from build123d import *

# Parameters (mm, degrees)
SKETCH1_W               = 110
SKETCH1_H               = 70
BOSS_EXTRUDE1_DEPTH     = 7
FILLET1_R               = 5
CUT_EXTRUDE1_DEPTH      = 40
SHELL1_START            = 5
SHELL1_DEPTH            = 2
SHELL1_START_2          = 2
SHELL1_2_DEPTH          = 3
SHELL1_START_3          = -42
SHELL1_3_DEPTH          = 40
SHELL1_4_DEPTH          = 2
SKETCH2_W               = 80
SKETCH2_H               = 0.8
SKETCH2_W_2             = 0.8
SKETCH2_H_2             = 40
BOSS_EXTRUDE2_DEPTH     = 6
CHAMFER1_SIZE           = 0.5
SKETCH8_R               = 4.15
BOSS_EXTRUDE3_DEPTH     = 3.2
CUT_EXTRUDE5_DEPTH      = 131.48770057
CUT_EXTRUDE5_DEPTH_BACK = 131.48770057
SKETCH9_R               = 1.5
SKETCH10_R              = 3
CUT_EXTRUDE6_DEPTH      = 3.2
CHAMFER2_SIZE           = 0.5
BOSS_EXTRUDE4_REACH     = 120.017


with BuildPart() as part:
    # Sketch1 → Boss-Extrude1 (new body)
    with BuildSketch(Plane(origin=(0, 0, 0), x_dir=(1, 0, 0), z_dir=(0, 1, 0))):
        with Locations((55, 35)):
            Rectangle(SKETCH1_W, SKETCH1_H)
    extrude(amount=BOSS_EXTRUDE1_DEPTH)

    # Fillet1
    fillet1_edges = [part.edges().sort_by_distance(p)[0] for p in [
        (0, 3.5, -70),
        (110, 3.5, -70),
        (110, 3.5, 0),
        (0, 3.5, 0),
    ]]
    fillet(fillet1_edges, radius=FILLET1_R)

    # Sketch3 → Cut-Extrude1 (cut)
    with BuildSketch(Plane.XY):
        Polygon((38, 0), (35, 3), (45, 3), (42, 0), align=None)
        Polygon((68, 0), (65, 3), (75, 3), (72, 0), align=None)
    extrude(amount=-CUT_EXTRUDE1_DEPTH, mode=Mode.SUBTRACT)

    # Shell1: read off the stored shape, not the designer's step
    # Shell1 outline → Shell1 (cut)
    with BuildSketch(Plane(origin=(0, 0, 0), x_dir=(1, 0, 0), z_dir=(0, 1, 0)).offset(SHELL1_START)):
        with BuildLine():
            Line((2, 65), (2, 5))
            ThreePointArc((2, 5), (2.878679656, 2.878679656), (5, 2))
            Line((5, 2), (105, 2))
            ThreePointArc((105, 2), (107.121320344, 2.878679656), (108, 5))
            Line((108, 5), (108, 65))
            ThreePointArc((108, 65), (107.121320344, 67.121320344), (105, 68))
            Line((105, 68), (5, 68))
            ThreePointArc((5, 68), (2.878679656, 67.121320344), (2, 65))
        make_face()
    extrude(amount=SHELL1_DEPTH, mode=Mode.SUBTRACT)

    # Shell1 2 outline → Shell1 2 (cut)
    with BuildSketch(Plane(origin=(0, 0, 0), x_dir=(1, 0, 0), z_dir=(0, 1, 0)).offset(SHELL1_START_2)):
        with BuildLine():
            Line((2, 65), (2, 5))
            ThreePointArc((2, 5), (2.878679656, 2.878679656), (5, 2))
            Line((5, 2), (105, 2))
            ThreePointArc((105, 2), (107.121320344, 2.878679656), (108, 5))
            Line((108, 5), (108, 65))
            ThreePointArc((108, 65), (107.121320344, 67.121320344), (105, 68))
            Line((105, 68), (5, 68))
            ThreePointArc((5, 68), (2.878679656, 67.121320344), (2, 65))
        make_face()
    extrude(amount=SHELL1_2_DEPTH, mode=Mode.SUBTRACT)

    # Shell1 3 outline → Shell1 3 (add)
    with BuildSketch(Plane.XY.offset(SHELL1_START_3)):
        Polygon((36, 2), (35, 3), (45, 3), (44, 2), (46.828427125, 2), (49.828427125, 5), (30.171572875, 5), (33.171572875, 2), align=None)
        Polygon((60.171572875, 5), (63.171572875, 2), (66, 2), (65, 3), (75, 3), (74, 2), (76.828427125, 2), (79.828427125, 5), align=None)
    extrude(amount=SHELL1_3_DEPTH)

    # Shell1 4 outline → Shell1 4 (add)
    with BuildSketch(Plane.XY.offset(SHELL1_START_3)):
        Polygon((45, 3), (35, 3), (36, 2), (44, 2), align=None)
        Polygon((65, 3), (66, 2), (74, 2), (75, 3), align=None)
    extrude(amount=SHELL1_4_DEPTH)

    # Sketch2 → Boss-Extrude2 (add)
    with BuildSketch(Plane(origin=(0, 2, 0), x_dir=(1, 0, 0), z_dir=(0, 1, 0))):
        with Locations((55, 67.6)):
            Rectangle(SKETCH2_W, SKETCH2_H)
        with Locations((107.6, 35)):
            Rectangle(SKETCH2_W_2, SKETCH2_H_2)
        with Locations((2.4, 35)):
            Rectangle(SKETCH2_W_2, SKETCH2_H_2)
    extrude(amount=BOSS_EXTRUDE2_DEPTH)

    # Chamfer1
    chamfer1_edges = [part.edges().sort_by_distance(p)[0] for p in [
        (55, 8, -68),
        (108, 8, -35),
        (2, 8, -35),
    ]]
    chamfer(chamfer1_edges, length=CHAMFER1_SIZE)

    # Sketch8 → Boss-Extrude3 (add)
    with BuildSketch(Plane(origin=(0, 2, 0), x_dir=(1, 0, 0), z_dir=(0, 1, 0))):
        with Locations((103.55, 64.85)):
            Circle(SKETCH8_R)
        with Locations((6.65, 64.85)):
            Circle(SKETCH8_R)
        with Locations((6.65, 4.15)):
            Circle(SKETCH8_R)
        with Locations((103.55, 4.15)):
            Circle(SKETCH8_R)
    extrude(amount=BOSS_EXTRUDE3_DEPTH)

    # Sketch9 → Cut-Extrude5 (cut, two sides: drawn at the far end of the back side and taken through both)
    with BuildSketch(Plane(origin=(0, 5.2, 0), x_dir=(1, 0, 0), z_dir=(0, 1, 0)).offset(-CUT_EXTRUDE5_DEPTH_BACK)):
        with Locations(Location((6.65, 64.85, 0), (0, 0, 270))):
            Circle(SKETCH9_R)
        with Locations(Location((6.65, 4.15, 0), (0, 0, 270))):
            Circle(SKETCH9_R)
        with Locations(Location((103.55, 4.15, 0), (0, 0, 270))):
            Circle(SKETCH9_R)
        with Locations(Location((103.55, 64.85, 0), (0, 0, 270))):
            Circle(SKETCH9_R)
    extrude(amount=CUT_EXTRUDE5_DEPTH + CUT_EXTRUDE5_DEPTH_BACK, mode=Mode.SUBTRACT)

    # Sketch10 → Cut-Extrude6 (cut)
    with BuildSketch(Plane(origin=(0, 0, 0), x_dir=(-1, 0, 0), z_dir=(0, -1, 0))):
        with Locations(Location((-6.65, 4.15, 0), (0, 0, 90))):
            Circle(SKETCH10_R)
        with Locations(Location((-6.65, 64.85, 0), (0, 0, 90))):
            Circle(SKETCH10_R)
        with Locations(Location((-103.55, 64.85, 0), (0, 0, 90))):
            Circle(SKETCH10_R)
        with Locations(Location((-103.55, 4.15, 0), (0, 0, 90))):
            Circle(SKETCH10_R)
    extrude(amount=-CUT_EXTRUDE6_DEPTH, mode=Mode.SUBTRACT)

    # Chamfer2
    chamfer2_edges = [part.edges().sort_by_distance(p)[0] for p in [
        (6.65, 0, -1.15),
        (6.65, 3.2, -5.65),
        (6.65, 0, -61.85),
        (6.65, 3.2, -66.35),
        (103.55, 0, -61.85),
        (103.55, 3.2, -66.35),
        (103.55, 0, -1.15),
        (103.55, 3.2, -5.65),
    ]]
    chamfer(chamfer2_edges, length=CHAMFER2_SIZE)

    # Sketch11 → Boss-Extrude4 (add, up to next)
    with BuildSketch(Plane(origin=(0, 0, -42), x_dir=(-1, 0, 0), z_dir=(0, 0, -1)), mode=Mode.PRIVATE) as boss_extrude4_sk1:
        Polygon((-60.171572875, 5), (-60.171572875, 2), (-63.171572875, 2), align=None)
    boss_extrude4_tool1 = extrude(boss_extrude4_sk1.sketch, amount=-BOSS_EXTRUDE4_REACH, mode=Mode.PRIVATE) - part.part
    # Sketch11 → Boss-Extrude4 (add, up to next)
    with BuildSketch(Plane(origin=(0, 0, -42), x_dir=(-1, 0, 0), z_dir=(0, 0, -1)), mode=Mode.PRIVATE) as boss_extrude4_sk2:
        Polygon((-49.828427125, 5), (-46.828427125, 2), (-49.828427125, 2), align=None)
    boss_extrude4_tool2 = extrude(boss_extrude4_sk2.sketch, amount=-BOSS_EXTRUDE4_REACH, mode=Mode.PRIVATE) - part.part
    # Sketch11 → Boss-Extrude4 (add, up to next)
    with BuildSketch(Plane(origin=(0, 0, -42), x_dir=(-1, 0, 0), z_dir=(0, 0, -1)), mode=Mode.PRIVATE) as boss_extrude4_sk3:
        Polygon((-33.171572875, 2), (-30.171572875, 5), (-30.171572875, 2), align=None)
    boss_extrude4_tool3 = extrude(boss_extrude4_sk3.sketch, amount=-BOSS_EXTRUDE4_REACH, mode=Mode.PRIVATE) - part.part
    # Sketch11 → Boss-Extrude4 (add, up to next)
    with BuildSketch(Plane(origin=(0, 0, -42), x_dir=(-1, 0, 0), z_dir=(0, 0, -1)), mode=Mode.PRIVATE) as boss_extrude4_sk4:
        Polygon((-79.828427125, 5), (-79.828427125, 2), (-76.828427125, 2), align=None)
    boss_extrude4_tool4 = extrude(boss_extrude4_sk4.sketch, amount=-BOSS_EXTRUDE4_REACH, mode=Mode.PRIVATE) - part.part
    add(boss_extrude4_tool1.solids().sort_by_distance((61.171573, 3, -42))[0])
    add(boss_extrude4_tool2.solids().sort_by_distance((48.828427, 3, -42))[0])
    add(boss_extrude4_tool3.solids().sort_by_distance((31.171573, 3, -42))[0])
    add(boss_extrude4_tool4.solids().sort_by_distance((78.828427, 3, -42))[0])


solid = part.part
Part model, mm, in its own coordinate system. A direction names the side the tool comes from. Give positions to 0.01 mm unless a question says otherwise; leave off trailing zeros. Loops run counter-clockwise (first coordinate to the right, second up) from the corner with the lowest first, then second, coordinate; pieces in that order, holes last. Notation, with made-up numbers: M 53.25,26 L 87.25,26 A19 cw 87.25,43 Z; hole C 58.25,69.5 d9. An arc over 180 degrees is marked long. Put each result on its own line as item: value. Start each with the question number.
1) Pull direction Z, two halves, no side cores. Call faces 1 (the cylindrical face through (102.8, 3.58, -8.23)), 2 (the flat face through (0, 3, -35)), 3 (the flat face through (54, 3, 0)): +Z half, -Z half, draft (parallel to the pull), parting line (faces both ways), or undercut.
2) Saw through at B-B (x = 18). List the corners of the cut face in (y, z), then the cut area to 3 significant figures.
3) Saw through at C-C (x = 6.65). State how many separate pieces and enclosed holes the cut face has, then the cut area to 3 significant figures.
4) 3-axis set-ups, long thin cutter, end or side, ignore diameter. For faces 4 (the flat face through (2, 4, -60)), 5 (the cylindrical face through (6.72, 4.44, -66.35)), 6 (the flat face through (104, 3.2, -2)): which of +Z, -Z, +X, -X, +Y, -Y reach the whole face in a straight line?
5) Saw through at D-D (z = -49). List the corners of the cut face in (x, y), then the cut area to 3 significant figures.
6) Probe probe 1 along X at (y, z) = (3.25, -38.5); probe 2 along Z at (x, y) = (103.55, 4.45); probe 3 along Z at (x, y) = (32, 3.5). List the from-to ranges inside material, lowest first.
7) Flat gauge pins, fed straight in: pin 1 (0.6 mm diameter, centred on x = 2.5, y = 4.5, fed in from -Z); pin 2 (5 mm diameter, centred on x = 6.65, z = -64.85, fed in from -Y); pin 3 (1 mm diameter, centred on x = 84, z = -61.5, fed in from +Y). Where does each tip first touch, or does it go through?
Numbers:
1. face 1: undercut
1. face 2: draft
1. face 3: +Z half
2. outline: M 0,-70 L 7,-70 L 7,-68 L 7.5,-68 L 8,-67.5 L 8,-67.2 L 2,-67.2 L 2,-2 L 7,-2 L 7,0 L 0,0 Z
2. area: 165 mm^2
3. separate pieces: 3
3. enclosed holes: 0
3. area: 152 mm^2
4. face 4: +Y
4. face 5: +Y, -Y
4. face 6: -Y
5. outline: M 0,0 L 110,0 L 110,7 L 108,7 L 108,7.5 L 107.5,8 L 107.2,8 L 107.2,2 L 2.8,2 L 2.8,8 L 2.5,8 L 2,7.5 L 2,7 L 0,7 Z
5. area: 249 mm^2
6. probe 1: 0 to 2.8, 30.17 to 49.83, 60.17 to 79.83, 107.2 to 110
6. probe 2: -70 to -66.35, -63.35 to -60.7, -8.3 to -5.65, -2.65 to 0
6. probe 3: -70 to -67.2, -42 to 0
7. pin 1: z = -69.49
7. pin 2: y = 3.2
7. pin 3: y = 2
